Here's how the part is built. I have some questions about the finished solid (model axes, mm). Coordinates: 2 decimals unless noted, no trailing zeros. Order: outer loops, then holes, each group sorted by start corner. A loop starts at its lowest first (then second) coordinate and runs counter-clockwise, first axis right, second up. Notation, with made-up numbers: (52, 77) - (59, 77) arc R13 cw to (59, 102) - close; hole circle Ø4 at (43.25, 22.25). An arc over 180 degrees is marked (long way). Answer in a Markdown table with one row per item. Add a question column.
Item 1: I want a section at D-D (x = -72). Please give me the cut outline in (y, z), plus the area to 3 significant figures.
Item 2: I want a section at B-B (x = 0). Please give me the cut outline in (y, z), plus the area to 3 significant figures.
Item 3: Will these pins go through, and if not, where does the flat tip stop? pin 1 Ø1.5 at (y, z) = (3.5, 37.5) entering from -X; pin 2 Ø1 at (y, z) = (2, 16) entering from -X; pin 3 Ø1.5 at (x, y) = (-39.5, 1.5) entering from +Z; pin 4 Ø8 at (x, z) = (0, 74.5) entering from -Y.
Item 4: I want a section at C-C (y = 0.8). Please give me the cut outline in (x, z).
Item 5: If I drill on line 1 along Z through (x, y) = (0, 3.05); line 2 along Z through (x, y) = (-5.5, 1.55); line 3 along Z through (x, y) = (-76.5, 0.8), over which ranges is the centre line in solid material (lowest first)? Write a range as from..to.
Item 6: I want a section at A-A (z = 0). Please give me the cut outline in (x, y).
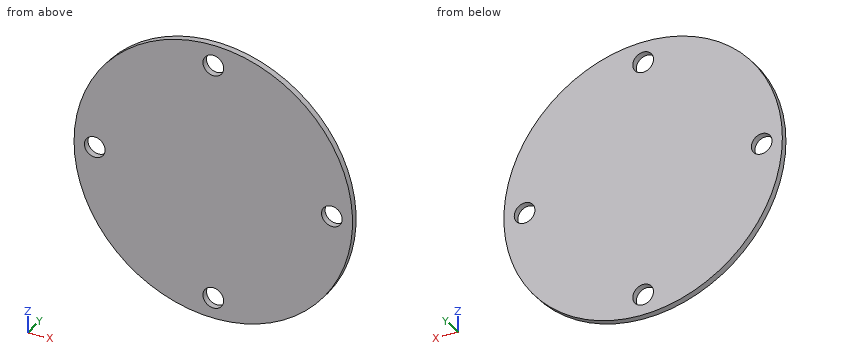
Autodesk Inventor part; units mm, degrees
ref_plane "YZ Plane" through (0, 0, 0) normal (1, 0, 0) x (0, 1, 0)
ref_plane "XZ Plane" through (0, 0, 0) normal (0, 1, 0) x (-1, 0, 0)
ref_plane "XY Plane" through (0, 0, 0) normal (0, 0, 1) x (1, 0, 0)
sketch "Sketch1" plane through (0, 0, 0) normal (0, 1, 0) x (-1, 0, 0)
  circle A0 centre (0, 0) radius 87.5
  dimension "d0" = 175
extrude "Plate1" add sketch "Sketch1" along normal blind 4
sketch "Sketch2" plane through (0, 4, 0) normal (0, 1, 0) x (1, 0, 0)
  line L0 (-40, -40) -> (40, -40) construction
  line L1 (40, -40) -> (40, 40) construction
  line L2 (40, 40) -> (-40, 40) construction
  line L3 (-40, 40) -> (-40, -40) construction
  line L4 (40, -40) -> (-40, 40) construction
  circle A0 centre (0, 0) radius 87.5
  line L5 (0, 0) -> (0, -87.5) construction
  circle A1 centre (0, -74.5) radius 6.5
  dimension "d2" = 80
  dimension "d3" = 80
  dimension "d16" = 13
  dimension "d23" = 74.5
extrude "Extrusion1" cut sketch "Sketch2" against normal through all contours A1
pattern_circular "Circular Pattern1" count 4 over 360 about axis through (0, -10, 0) along (0, 1, 0) of "Extrusion1"
sketch "Sketch3" plane through (0, 4, 0) normal (0, 1, 0) x (1, 0, 0)
  line L0 (9.823, 55.7091) -> (-55.7091, 9.823)
  line L1 (-55.7091, 9.823) -> (-9.823, -55.7091)
  line L2 (-9.823, -55.7091) -> (55.7091, -9.823)
  line L3 (55.7091, -9.823) -> (9.823, 55.7091) construction
  line L4 (32.7661, 22.9431) -> (-32.7661, -22.9431) construction
  line L5 (0, 0) -> (26.1739, 0) construction
  line L6 (-55.7091, -9.823) -> (9.823, -55.7091)
  line L7 (9.823, -55.7091) -> (55.7091, 9.823)
  line L8 (55.7091, 9.823) -> (-9.823, 55.7091) construction
  line L9 (-9.823, 55.7091) -> (-55.7091, -9.823)
  line L10 (22.9431, 32.7661) -> (-22.9431, -32.7661)
  line L11 (9.823, -55.7091) -> (39.823, -55.7091)
  line L12 (-55.7091, 9.823) -> (-55.7091, 39.823)
  dimension "d18" = 80
  dimension "d19" = 35
  dimension "d20" = 55
  dimension "d21" = 30
  dimension "d22" = 30
mark "Mark1"
equation "\"d1\" = Thickness"
equation "\"BendReliefWidth\" = Thickness"
equation "\"BendReliefDepth\" = 0.5 * Thickness"
equation "\"CornerReliefSize\" = 4 * Thickness"
equation "\"MinimumRemnant\" = 2 * Thickness"
equation "\"TransitionRadius\" = BendRadius"
equation "\"JacobiRadiusSize\" = BendRadius"
equation "\"GapSize\" = Thickness"
properties part number "MSC 904 FLANGE BASE TUBE" material "Stainless Steel"
Values follow:
| question | item | result |
|---|---|---|
| 1 | outline | (0, -49.72) - (4, -49.72) - (4, -6) - (0, -6) - close; (0, 6) - (4, 6) - (4, 49.72) - (0, 49.72) - close |
| 1 | area | 350 mm^2 |
| 2 | outline | (0, -87.5) - (4, -87.5) - (4, -81) - (0, -81) - close; (0, -68) - (4, -68) - (4, 68) - (0, 68) - close; (0, 81) - (4, 81) - (4, 87.5) - (0, 87.5) - close |
| 2 | area | 596 mm^2 |
| 3 | pin 1 | stops at x = -79.41 |
| 3 | pin 2 | stops at x = -86.12 |
| 3 | pin 3 | stops at z = 78.45 |
| 3 | pin 4 | passes through |
| 4 | outline | circle Ø175 at (0, 0); hole circle Ø13 at (-74.5, 0); hole circle Ø13 at (0, -74.5); hole circle Ø13 at (0, 74.5); hole circle Ø13 at (74.5, 0) |
| 5 | line 1 | z = -87.5..-81, -68..68, 81..87.5 |
| 5 | line 2 | z = -87.33..-77.96, -71.04..71.04, 77.96..87.33 |
| 5 | line 3 | z = -42.47..-6.18, 6.18..42.47 |
| 6 | outline | (-87.5, 0) - (-81, 0) - (-81, 4) - (-87.5, 4) - close; (-68, 0) - (68, 0) - (68, 4) - (-68, 4) - close; (81, 0) - (87.5, 0) - (87.5, 4) - (81, 4) - close |
